```python
from build123d import *

# Parameters (mm, degrees)
SKETCH_1_W          = 10
SKETCH_1_H          = 10
SKETCH_1_W_2        = 8
SKETCH_1_H_2        = 8
EXTRUDE_1_DEPTH     = 30
SKETCH_3_R          = 1.6
CUT_EXTRUDE_1_DEPTH = 11
SKETCH_4_R          = 1.6
CUT_EXTRUDE_2_DEPTH = 11


with BuildPart() as part:
    # ｽｹｯﾁ1 → ﾎﾞｽ - 押し出し1 (new body, symmetric)
    with BuildSketch(Plane.XY):
        Rectangle(SKETCH_1_W, SKETCH_1_H)
        Rectangle(SKETCH_1_W_2, SKETCH_1_H_2, mode=Mode.SUBTRACT)
    extrude(amount=EXTRUDE_1_DEPTH, both=True)

    # ｽｹｯﾁ3 → ｶｯﾄ - 押し出し1 (cut, through all)
    with BuildSketch(Plane(origin=(5, 0, 0), x_dir=(0, 0, -1), z_dir=(1, 0, 0))):
        with Locations((-25, 0)):
            Circle(SKETCH_3_R)
        with Locations((25, 0)):
            Circle(SKETCH_3_R)
    extrude(amount=-CUT_EXTRUDE_1_DEPTH, mode=Mode.SUBTRACT)

    # ｽｹｯﾁ4 → ｶｯﾄ - 押し出し2 (cut, through all)
    with BuildSketch(Plane(origin=(0, 5, 0), x_dir=(1, 0, 0), z_dir=(0, 1, 0))):
        with Locations((0, -20)):
            Circle(SKETCH_4_R)
        with Locations((0, 20)):
            Circle(SKETCH_4_R)
    extrude(amount=-CUT_EXTRUDE_2_DEPTH, mode=Mode.SUBTRACT)


solid = part.part
```
Part model, mm, in its own coordinate system. A direction names the side the tool comes from. Coordinates: 2 decimals unless noted, no trailing zeros. Write each loop counter-clockwise with the first axis right and the second up, starting at its lowest first coordinate (ties: lowest second). Pieces come first, ordered by that corner, then holes.
Item 1: Pin check, flat tip, straight feed: pin 1 (3 mm diameter, centred on x = 0, z = 20, fed in from +Y). Stop position of the tip, or through.
Item 2: Mould opens along Y. For faces 1 (the face through (0, -5, 0)), 2 (the face through (4.51, 1.08, 26.18)), 3 (the face through (0, 5, 0)), 4 (the face through (-5, 0, 0)) say: released by +Y, released by -Y, zero draft, split by the parting line, or undercut.
Item 3: Slice it at D-D (z = -20). Write the cut outline in (x, y), and give its area (3 significant figures).
Item 4: Which spindle directions (+Z, -Z, +X, -X, +Y, -Y) get a long thin tool onto all of the face, cutting with end or side? Do faces 5 (the face through (4, 0, 0)), 6 (the face through (-0.208, 4.507, -21.586)). Say none if no direction does.
Item 5: Slice it at B-B (x = 3). Write the cut outline in (y, z).
Item 6: Slice it at A-A (y = 0). Write the cut outline in (x, z), and give its area (3 significant figures).
Item 7: Probe line 1 (Z direction, x = 0, y = 4.5); line 2 (Y direction, x = 3.5, z = -5.5); line 3 (Y direction, x = 4.4, z = 25). List the from-to ranges inside material, lowest first.
Results found:
1. pin 1: passes through
2. face 1: released by -Y
2. face 2: undercut
2. face 3: released by +Y
2. face 4: zero draft
3. outline: (-5, -5) - (-1.6, -5) - (-1.6, -4) - (-4, -4) - (-4, 4) - (-1.6, 4) - (-1.6, 5) - (-5, 5) - close; (1.6, -5) - (5, -5) - (5, 5) - (1.6, 5) - (1.6, 4) - (4, 4) - (4, -4) - (1.6, -4) - close
3. area: 29.6 mm2
4. face 5: +Z, -Z
4. face 6: +Y, -Y
5. outline: (-5, -30) - (-4, -30) - (-4, 30) - (-5, 30) - close; (4, -30) - (5, -30) - (5, 30) - (4, 30) - close
6. outline: (-5, -30) - (-4, -30) - (-4, -26.6) - (-5, -26.6) - close; (-5, -23.4) - (-4, -23.4) - (-4, 23.4) - (-5, 23.4) - close; (-5, 26.6) - (-4, 26.6) - (-4, 30) - (-5, 30) - close; (4, -30) - (5, -30) - (5, -26.6) - (4, -26.6) - close; (4, -23.4) - (5, -23.4) - (5, 23.4) - (4, 23.4) - close; (4, 26.6) - (5, 26.6) - (5, 30) - (4, 30) - close
6. area: 107 mm2
7. line 1: z = -30 to -21.6, -18.4 to 18.4, 21.6 to 30
7. line 2: y = -5 to -4, 4 to 5
7. line 3: y = -5 to -1.6, 1.6 to 5
